Autodesk Inventor part; units mm, degrees
ref_plane "YZ Plane" through (0, 0, 0) normal (1, 0, 0) x (0, 1, 0)
ref_plane "XZ Plane" through (0, 0, 0) normal (0, 1, 0) x (-1, 0, 0)
ref_plane "XY Plane" through (0, 0, 0) normal (0, 0, 1) x (1, 0, 0)
sketch "Block1" plane through (0, 0, 0) normal (0, 0, 1) x (1, 0, 0)
  circle A0 centre (0, 0) radius 40.22
  circle A1 centre (30, -0.0076) radius 2.22
  circle A2 centre (0.0076, 30) radius 2.22
  circle A3 centre (0, 0) radius 5.22
  circle A4 centre (-30, 0.0076) radius 2.22
  circle A5 centre (-0.0076, -30) radius 2.22
  point P0 (0, 0)
sketch "Block2" plane through (0, 0, 0) normal (0, 0, 1) x (1, 0, 0)
  circle A0 centre (0, 0) radius 20.22
  circle A1 centre (10, -0.0076) radius 2.22
  circle A2 centre (0.0076, 10) radius 2.22
  circle A3 centre (0, 0) radius 5.22
  circle A4 centre (-0.0076, -10) radius 2.22
  circle A5 centre (-10, 0.0076) radius 2.22
  point P0 (0, 0)
sketch "Block3" plane through (0, 0, 0) normal (0, 0, 1) x (1, 0, 0)
  line L0 (-21.2132, 8.22) -> (21.2132, 8.22)
  arc A0 (21.2132, -8.22) -> (21.2132, 8.22) centre (21.2132, 0) ccw
  line L1 (21.2132, -8.22) -> (-21.2132, -8.22)
  arc A1 (-21.2132, 8.22) -> (-21.2132, -8.22) centre (-21.2132, 0) ccw
  circle A2 centre (0, 0) radius 5.22
  circle A3 centre (-21.2132, 0) radius 2.72
  circle A4 centre (21.2132, 0) radius 2.72
  point P0 (0, 0)
sketch "Sketch1" plane through (0, 0, 0) normal (0, 1, 0) x (-1, 0, 0)
  circle A0 centre (0, 0) radius 30
  circle A1 centre (0, 0) radius 5
  arc A2 (-36.0813, 0.572) -> (-36.0815, -0.5576) centre (0, 0) ccw
  arc A3 (-0.0152, -40) -> (-0.0008, -40) centre (0, 0) ccw
  arc A4 (-0.5728, -36.0815) -> (0.5584, -36.0818) centre (0, 0) ccw
  circle A5 centre (15, 15) radius 2.5
  line L0 (43.2172, 0) -> (-49.3032, 0)
  line L1 (0, -55.2163) -> (0, 51.2978)
  circle A6 centre (15, -15) radius 2.5
  circle A7 centre (-15, 15) radius 2.5
  circle A8 centre (-15, -15) radius 2.5
  point P0 (17, -0.0008)
  point P1 (13.0813, -0.572)
  point P2 (-36.0815, 0.5728)
  point P3 (-0.5576, 36.0815)
  point P4 (0.572, 36.0813)
  point P5 (-13.0813, -0.572)
  dimension "d0" = 60
  dimension "d7" = 10
  dimension "d31" = 5
  dimension "d32" = 15
  dimension "d33" = 15
ref_plane "Work Plane1" through (0, 10, 0) normal (0, 1, 0) x (1, 0, 0)
sketch "Sketch6" plane through (0, 0, 0) normal (0, 1, 0) x (-1, 0, 0)
  line L0 (21.2132, 0) -> (-21.2132, 0) construction
  line L1 (21.2132, 8) -> (-21.2132, 8)
  line L2 (-21.2132, -8) -> (21.2132, -8)
  arc A0 (21.2132, -8) -> (21.2132, 8) centre (21.2132, 0) ccw
  arc A1 (-21.2132, 8) -> (-21.2132, -8) centre (-21.2132, 0) ccw
  circle A2 centre (-21.2132, 0) radius 2.5
  circle A3 centre (21.2132, 0) radius 2.5
  circle A4 centre (0, 0) radius 5
  dimension "d36" = 8
  dimension "d37" = 5
  dimension "d38" = 5
  dimension "d39" = 42.4264
  dimension "d40" = 10
extrude "Extrusion4" add sketch "Sketch6" along normal blind 10
sketch "Sketch7" plane through (21.2132, 0, -8) normal (0, 0, -1) x (-1, 0, 0)
  circle A0 centre (21.2132, 5) radius 2.5
  line L0 (0, 10) -> (42.4264, 10)
  line L1 (0, 0) -> (0, 10)
  point P0 (21.2132, 0)
  dimension "d43" = 5
  dimension "d44" = 5
  dimension "d45" = 21.2132
extrude "Extrusion5" cut sketch "Sketch7" against normal through all
sketch "Sketch8" plane through (0, 10, 0) normal (0, 1, 0) x (1, 0, 0)
  circle A0 centre (0, 0) radius 5
  circle A1 centre (-21.2132, 0) radius 2.5
  circle A2 centre (21.2132, 0) radius 2.5
  line L0 (-21.2132, -8) -> (21.2132, -8)
  arc A3 (21.2132, -8) -> (21.2132, 8) centre (21.2132, 0) ccw
  line L1 (21.2132, 8) -> (-21.2132, 8)
  arc A4 (-21.2132, 8) -> (-21.2132, -8) centre (-21.2132, 0) ccw
sketch "DXF" plane through (0, 0, 0) normal (0, 1, 0) x (-1, 0, 0)
  point P0 (0, 0)
properties part number "pulleyFlange"
Input: part model. Units: mm. Frame: model coordinates. Give positions to 0.01 mm unless a question says otherwise; leave off trailing zeros. Order: outer loops, then holes, each group sorted by start corner. A loop starts at its lowest first (then second) coordinate and runs counter-clockwise, first axis right, second up. Notation, with made-up numbers: (25.25, 86) -> (48.25, 86) arc R16 cw to (48.25, 113) -> close; hole circle Ø4 at (88.25, 41). An arc over 180 degrees is marked (long way). Write each question's results on one line, items separated by ' | '. Start each with the question number.
Item 1: Contact query for flat-ended pins moving along their axis: P1, Ø8, axis at x = 21.21, z = 0, coming from the +Y side; P2, Ø5, axis at y = 6, z = -4.5, coming from the +X side; P3, Ø1.5, axis at y = 2, z = -1, coming from the -X side. Output: stop coordinate, or through.
Item 2: Cut plane B-B on z = 0. Return the cut outline in (x, y).
Item 3: Cut plane A-A on x = 0. Return the cut outline in (y, z).
Item 4: Line query: line 1 (X direction, y = 7.5, z = 1); line 2 (Z direction, x = 21, y = 1.75); line 3 (Y direction, x = 0, z = 5.4). Output: solid intervals per line, ascending.
Item 5: Mould query, pull axis X, two halves, no side actions, for faces 1 (the cylindrical face through (-4.619, 4.93, 1.915)), 2 (the cylindrical face through (29.21, 4.93, -0.18)), 3 (the flat face through (0, 2, 8)). Classes: pulls with the +X half, pulls with the -X half, needs draft (parallel to the pull), parting line crosses it, or undercut.
Item 6: Cut plane C-C on y = 5. Return the cut outline in (x, z), then the cut area to 3 significant figures.
Item 7: Cut plane D-D on z = -6.25. Return the cut outline in (x, y), then the cut area to 3 significant figures.
Established:
1) P1: y = 10 | P2: x = 28.96 | P3: x = -29.21
2) outline: (-29.21, 0) -> (-23.71, 0) -> (-23.71, 10) -> (-29.21, 10) -> close; (-18.71, 0) -> (-5, 0) -> (-5, 10) -> (-18.71, 10) -> close; (5, 0) -> (18.71, 0) -> (18.71, 10) -> (5, 10) -> close; (23.71, 0) -> (29.21, 0) -> (29.21, 10) -> (23.71, 10) -> close
3) outline: (0, -8) -> (2.5, -8) -> (2.5, -5) -> (0, -5) -> close; (0, 5) -> (2.5, 5) -> (2.5, 8) -> (0, 8) -> close; (7.5, -8) -> (10, -8) -> (10, -5) -> (7.5, -5) -> close; (7.5, 5) -> (10, 5) -> (10, 8) -> (7.5, 8) -> close
4) line 1: -29.15 to -23.5, -18.92 to -4.9, 4.9 to 18.92, 23.5 to 29.15 | line 2: -8 to -2.49, 2.49 to 8 | line 3: 0 to 2.5, 7.5 to 10
5) face 1: undercut | face 2: pulls with the +X half | face 3: needs draft
6) outline: (-21.21, -8) -> (-2.5, -8) -> (-2.5, -4.33) arc R5 cw to (-2.5, 4.33) -> (-2.5, 8) -> (-21.21, 8) arc R8 ccw to start; (2.5, -8) -> (21.21, -8) arc R8 ccw to (21.21, 8) -> (2.5, 8) -> (2.5, 4.33) arc R5 cw to (2.5, -4.33) -> close; hole circle Ø5 at (-21.21, 0); hole circle Ø5 at (21.21, 0) | area: 730 mm^2
7) outline: (-26.21, 0) -> (26.21, 0) -> (26.21, 10) -> (-26.21, 10) -> close; hole circle Ø5 at (0, 5) | area: 505 mm^2
